from build123d import *

# Parameters (mm, degrees)
CROQUIS1_R              = 4.05
SALIENTE_EXTRUIR1_DEPTH = 12
CORTAR_EXTRUIR1_REACH   = 8
CROQUIS2_R              = 1.5
REDONDEO1_R             = 0.5
REDONDEO2_R             = 0.1


with BuildPart() as part:
    # Croquis1 → Saliente-Extruir1 (new body, symmetric)
    with BuildSketch(Plane.XY):
        with BuildLine():
            Line((15, 0), (-15, 0))
            Line((-15, 0), (-15, 6))
            Line((-15, 6), (-8.1, 6))
            Line((-8.1, 6), (-8.1, 10))
            ThreePointArc((-8.1, 10), (0, 18.1), (8.1, 10))
            Line((8.1, 10), (8.1, 6))
            Line((8.1, 6), (15, 6))
            Line((15, 6), (15, 0))
        make_face()
        with Locations((0, 10)):
            Circle(CROQUIS1_R, mode=Mode.SUBTRACT)
    extrude(amount=SALIENTE_EXTRUIR1_DEPTH, both=True)

    # Croquis2 → Cortar-Extruir1 (cut, up to next)
    with BuildSketch(Plane(origin=(0, 6, 0), x_dir=(1, 0, 0), z_dir=(0, 1, 0)), mode=Mode.PRIVATE) as cortar_extruir1_sk1:
        with Locations((-12, 9)):
            Circle(CROQUIS2_R)
    cortar_extruir1_tool1 = extrude(cortar_extruir1_sk1.sketch, amount=-CORTAR_EXTRUIR1_REACH, mode=Mode.PRIVATE) & part.part
    add(cortar_extruir1_tool1.solids().sort_by_distance((-12, 6, -9))[0], mode=Mode.SUBTRACT)
    # Croquis2 → Cortar-Extruir1 (cut, up to next)
    with BuildSketch(Plane(origin=(0, 6, 0), x_dir=(1, 0, 0), z_dir=(0, 1, 0)), mode=Mode.PRIVATE) as cortar_extruir1_sk2:
        with Locations((12, 9)):
            Circle(CROQUIS2_R)
    cortar_extruir1_tool2 = extrude(cortar_extruir1_sk2.sketch, amount=-CORTAR_EXTRUIR1_REACH, mode=Mode.PRIVATE) & part.part
    add(cortar_extruir1_tool2.solids().sort_by_distance((12, 6, -9))[0], mode=Mode.SUBTRACT)
    # Croquis2 → Cortar-Extruir1 (cut, up to next)
    with BuildSketch(Plane(origin=(0, 6, 0), x_dir=(1, 0, 0), z_dir=(0, 1, 0)), mode=Mode.PRIVATE) as cortar_extruir1_sk3:
        with Locations((-12, -9)):
            Circle(CROQUIS2_R)
    cortar_extruir1_tool3 = extrude(cortar_extruir1_sk3.sketch, amount=-CORTAR_EXTRUIR1_REACH, mode=Mode.PRIVATE) & part.part
    add(cortar_extruir1_tool3.solids().sort_by_distance((-12, 6, 9))[0], mode=Mode.SUBTRACT)
    # Croquis2 → Cortar-Extruir1 (cut, up to next)
    with BuildSketch(Plane(origin=(0, 6, 0), x_dir=(1, 0, 0), z_dir=(0, 1, 0)), mode=Mode.PRIVATE) as cortar_extruir1_sk4:
        with Locations((12, -9)):
            Circle(CROQUIS2_R)
    cortar_extruir1_tool4 = extrude(cortar_extruir1_sk4.sketch, amount=-CORTAR_EXTRUIR1_REACH, mode=Mode.PRIVATE) & part.part
    add(cortar_extruir1_tool4.solids().sort_by_distance((12, 6, 9))[0], mode=Mode.SUBTRACT)

    # Redondeo1
    redondeo1_edges = [part.edges().sort_by_distance(p)[0] for p in [
        (8.1, 8, -12),
        (11.55, 6, 12),
        (15, 3, 12),
        (-15, 3, 12),
        (-11.55, 6, 12),
        (-8.1, 8, 12),
        (0, 18.1, 12),
        (8.1, 8, 12),
        (0, 18.1, -12),
        (8.1, 6, 0),
        (15, 6, 0),
        (-15, 6, 0),
        (-8.1, 6, 0),
        (-8.1, 8, -12),
        (-11.55, 6, -12),
        (-15, 3, -12),
        (15, 3, -12),
        (11.55, 6, -12),
    ]]
    fillet(redondeo1_edges, radius=REDONDEO1_R)

    # Redondeo2
    redondeo2_edges = [part.edges().sort_by_distance(p)[0] for p in [
        (-4.05, 10, 12),
        (-4.05, 10, -12),
    ]]
    fillet(redondeo2_edges, radius=REDONDEO2_R)


solid = part.part
Could you check a few things on this model? Use its own coordinates, in mm. A direction names the side the tool comes from. Coordinates: 2 decimals unless noted, no trailing zeros. Write each loop counter-clockwise with the first axis right and the second up, starting at its lowest first coordinate (ties: lowest second). Pieces come first, ordered by that corner, then holes. Notation, with made-up numbers: (75.25, -33) - (113.25, -33) arc R11 cw to (113.25, -17) - close; hole circle Ø7 at (26.25, 61.5). An arc over 180 degrees is marked (long way). Write item = value, one per line.
1) Suppose I cut it at C-C on x = 0. Please give me the cut outline in (y, z).
Result set:
outline = (0, -12) - (5.85, -12) arc R0.1 ccw to (5.95, -11.9) - (5.95, 11.9) arc R0.1 ccw to (5.85, 12) - (0, 12) - close; (14.05, -11.9) arc R0.1 ccw to (14.15, -12) - (17.6, -12) arc R0.5 ccw to (18.1, -11.5) - (18.1, 11.5) arc R0.5 ccw to (17.6, 12) - (14.15, 12) arc R0.1 ccw to (14.05, 11.9) - close
2) Will these pins go through, and if not, where does the flat tip stop? pin 1 Ø1.8 at (x, z) = (11, 3.5) entering from +Y; pin 2 Ø6 at (y, z) = (15, -8.5) entering from -X; pin 3 Ø3 at (y, z) = (15, 3.5) entering from +X.
Result set:
pin_1 = 6
pin_2 = -7.85
pin_3 = 7.3
3) Please list where these lines run through material, in increasing order: line 1 (X direction, y = 3.8, z = -9); line 2 (Z direction, x = -12, y = 1.6); line 3 (Y direction, x = 0, z = -2.25). Write a range as [from, to].
Result set:
line_1 = [-15, -13.5], [-10.5, 10.5], [13.5, 15]
line_2 = [-12, -10.5], [-7.5, 7.5], [10.5, 12]
line_3 = [0, 5.95], [14.05, 18.1]
4) Suppose I cut it at D-D on z = 3. Please give me the cut outline in (x, y), plus the area to 3 significant figures.
Result set:
outline = (-15, 0) - (15, 0) - (15, 5.5) arc R0.5 ccw to (14.5, 6) - (8.6, 6) arc R0.5 cw to (8.1, 6.5) - (8.1, 10) arc R8.1 ccw to (-8.1, 10) - (-8.1, 6.5) arc R0.5 cw to (-8.6, 6) - (-14.5, 6) arc R0.5 ccw to (-15, 5.5) - close; hole circle Ø8.1 at (0, 10)
area = 296 mm2
5) Suppose I cut it at B-B on z = 8. Please give me the cut outline in (x, y), plus the area to 3 significant figures.
Result set:
outline = (-15, 0) - (-13.12, 0) - (-13.12, 6) - (-14.5, 6) arc R0.5 ccw to (-15, 5.5) - close; (-10.88, 0) - (10.88, 0) - (10.88, 6) - (8.6, 6) arc R0.5 cw to (8.1, 6.5) - (8.1, 10) arc R8.1 ccw to (-8.1, 10) - (-8.1, 6.5) arc R0.5 cw to (-8.6, 6) - (-10.88, 6) - close; (13.12, 0) - (15, 0) - (15, 5.5) arc R0.5 ccw to (14.5, 6) - (13.12, 6) - close; hole circle Ø8.1 at (0, 10)
area = 269 mm2
6) We'd pull the mould along Y, two halves only. Please class faces 1 (the cylindrical face through (-0.878, 6.046, -0.167)), 2 (the flat face through (-12, 6, 0)), 3 (the flat face through (0, 5, -12)): +Y half, -Y half, draft (parallel to the pull), parting line (faces both ways), or undercut.
Result set:
face_1 = undercut
face_2 = +Y half
face_3 = draft
7) For faces 4 (the flat face through (-8.1, 8, 0)), 5 (the flat face through (12, 6, 0)), 6 (the flat face through (15, 3, 0)), which set-ups out of +Z, -Z, +X, -X, +Y, -Y let a thin tool reach every point of the face, with its end or its side?
Result set:
face_4 = +Z, -Z, -X, +Y
face_5 = +Z, -Z, +X, +Y
face_6 = +Z, -Z, +X, +Y, -Y
8) Suppose I cut it at A-A on x = 12. Please give me the cut outline in (y, z), plus the area to 3 significant figures.
Result set:
outline = (0, -12) - (5.5, -12) arc R0.5 ccw to (6, -11.5) - (6, -10.5) - (0, -10.5) - close; (0, -7.5) - (6, -7.5) - (6, 7.5) - (0, 7.5) - close; (0, 10.5) - (6, 10.5) - (6, 11.5) arc R0.5 ccw to (5.5, 12) - (0, 12) - close
area = 108 mm2
